Part model, mm, in its own coordinate system. Round coordinates to 2 decimals unless told otherwise and drop trailing zeros. Order: outer loops, then holes, each group sorted by start corner. A loop starts at its lowest first (then second) coordinate and runs counter-clockwise, first axis right, second up. Notation, with made-up numbers: M -31,-23.75 L 13,-23.75 A24 ccw 13,9.25 Z; hole C -9.5,39.25 d4. An arc over 180 degrees is marked long. One line per question, with ' | ' between items.
from build123d import *

# Parameters (mm, degrees)
BOSS_EXTRUDE1_DEPTH = 3.175
SKETCH3_R           = 3.175
CUT_EXTRUDE1_DEPTH  = 58.589283942


with BuildPart() as part:
    # Sketch2 → Boss-Extrude1 (new body)
    with BuildSketch(Plane.XY):
        with BuildLine():
            Line((-50.8, 6.35), (50.8, 6.35))
            ThreePointArc((50.8, 6.35), (57.15, 0), (50.8, -6.35))
            Line((50.8, -6.35), (-50.8, -6.35))
            ThreePointArc((-50.8, -6.35), (-57.15, 0), (-50.8, 6.35))
        make_face()
    extrude(amount=BOSS_EXTRUDE1_DEPTH)

    # Sketch3 → Cut-Extrude1 (cut, through all)
    with BuildSketch(Plane.XY.offset(3.175)):
        with Locations((-50.8, 0)):
            Circle(SKETCH3_R)
        with Locations(Location((50.8, 0, 0), (0, 0, 180))):
            Circle(SKETCH3_R)
    extrude(amount=-CUT_EXTRUDE1_DEPTH, mode=Mode.SUBTRACT)


solid = part.part
1) Two-plate mould, pull along Y, no slides. Class faces 1 (the face through (1, 0, 3.175)), 2 (the face through (-53.97, 0.14, 1.61)), 3 (the face through (1, -6.35, 2)): released by +Y, released by -Y, zero draft, split by the parting line, or undercut.
The answers:
face 1: zero draft | face 2: undercut | face 3: released by -Y
2) Saw through at A-A (y = 0). List the corners of the cut face in (x, z) (3 decimals).
The answers:
outline: M -57.15,0 L -53.975,0 L -53.975,3.175 L -57.15,3.175 Z; M -47.625,0 L 47.625,0 L 47.625,3.175 L -47.625,3.175 Z; M 53.975,0 L 57.15,0 L 57.15,3.175 L 53.975,3.175 Z
3) Drop a flat-ended pin along its axis: pin 1 (4 mm diameter, centred on x = 12, y = 2.5, fed in from -Z). Give the stop position or say it passes through.
The answers:
pin 1: stops at z = 0
4) Probe line 1 (Y direction, x = -50.8, z = 1.35) (3 decimals); line 2 (X direction, y = 2.5, z = 2.45). List the from-to ranges inside material, lowest first. Write a range as [from, to].
The answers:
line 1: y = [-6.35, -3.175], [3.175, 6.35] | line 2: x = [-56.64, -52.76], [-48.84, 48.84], [52.76, 56.64]
5) Saw through at C-C (y = -4.75). List the corners of the cut face in (x, z) (3 decimals), plus the area to 3 significant figures.
The answers:
outline: M -55.014,0 L 55.014,0 L 55.014,3.175 L -55.014,3.175 Z | area: 349 mm²
6) Saw through at B-B (z = 1.5). List the corners of the cut face in (x, y) (3 decimals).
The answers:
outline: M -50.8,-6.35 L 50.8,-6.35 A6.35 ccw 50.8,6.35 L -50.8,6.35 A6.35 ccw Z; hole C -50.8,0 d6.35; hole C 50.8,0 d6.35
